Build history of the part. All positions in model axes, mm. Face numbers are marked on the shaded views. A direction names the side the tool comes from. Coordinates: 2 decimals unless noted, no trailing zeros. Order: outer loops, then holes, each group sorted by start corner. A loop starts at its lowest first (then second) coordinate and runs counter-clockwise, first axis right, second up. Notation, with made-up numbers: (81, 47.5) - (131, 47.5) arc R10 ccw to (131, 54.5) - close; hole circle Ø7 at (18.5, -19.75). An arc over 180 degrees is marked (long way). Answer as CSV lines item,"result". Start each with the question number.
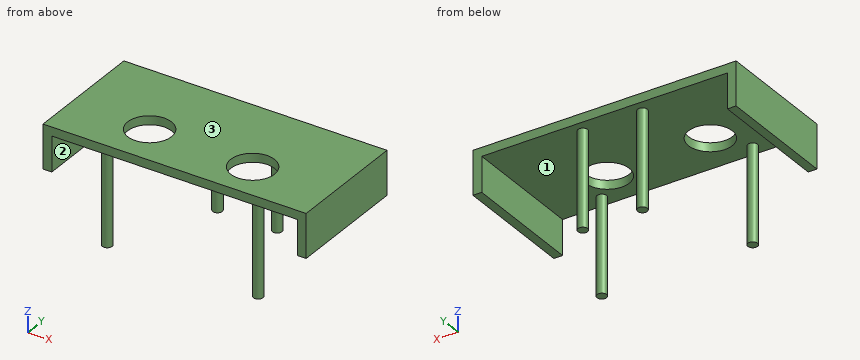
from build123d import *

# Parameters (mm, degrees)
ESQUISSE1_W             = 100
ESQUISSE1_H             = 69.87
BOSS_EXTRU_1_DEPTH      = 5
ESQUISSE2_R             = 12.5
ENL_V_MAT_EXTRU_1_DEPTH = 5
ESQUISSE3_W             = 25
ESQUISSE3_H             = 69.87
BOSS_EXTRU_2_DEPTH      = 5
ESQUISSE4_W             = 5
ESQUISSE4_H             = 69.87
BOSS_EXTRU_3_DEPTH      = 20
ESQUISSE2_3_R           = 2.75
BOSS_EXTRU_4_DEPTH      = 60
ESQUISSE2_4_R           = 2.75
BOSS_EXTRU_5_DEPTH      = 60
ESQUISSE2_5_R           = 2.75
BOSS_EXTRU_6_DEPTH      = 60
ESQUISSE2_6_R           = 2.75
BOSS_EXTRU_7_DEPTH      = 60


with BuildPart() as part:
    # Esquisse1 → Boss.-Extru.1 (new body)
    with BuildSketch(Plane.XY):
        with Locations((-50, 34.935)):
            Rectangle(ESQUISSE1_W, ESQUISSE1_H)
    extrude(amount=BOSS_EXTRU_1_DEPTH)

    # Esquisse2 → Enlèv. mat.-Extru.1 (cut)
    with BuildSketch(Plane.XY.offset(5)):
        with Locations((-80, 23.913092396)):
            Circle(ESQUISSE2_R)
        with Locations((-20, 21.980812212)):
            Circle(ESQUISSE2_R)
    extrude(amount=-ENL_V_MAT_EXTRU_1_DEPTH, mode=Mode.SUBTRACT)

    # Esquisse3 → Boss.-Extru.2 (add)
    with BuildSketch(Plane.XY.offset(5)):
        with Locations((-112.5, 34.935)):
            Rectangle(ESQUISSE3_W, ESQUISSE3_H)
        with Locations((12.5, 34.935)):
            Rectangle(ESQUISSE3_W, ESQUISSE3_H)
    extrude(amount=-BOSS_EXTRU_2_DEPTH)

    # Esquisse4 → Boss.-Extru.3 (add)
    with BuildSketch(Plane(origin=(0, 0, 0), x_dir=(-1, 0, 0), z_dir=(0, 0, -1))):
        with Locations((122.5, 34.935)):
            Rectangle(ESQUISSE4_W, ESQUISSE4_H)
        with Locations((-22.5, 34.935)):
            Rectangle(ESQUISSE4_W, ESQUISSE4_H)
    extrude(amount=BOSS_EXTRU_3_DEPTH)

    # Esquisse2<3> → Boss.-Extru.4 (add)
    with BuildSketch(Plane.XY.offset(5)):
        with Locations((-67, 62.87)):
            Circle(ESQUISSE2_3_R)
    extrude(amount=-BOSS_EXTRU_4_DEPTH)

    # Esquisse2<4> → Boss.-Extru.5 (add)
    with BuildSketch(Plane.XY.offset(5)):
        with Locations((-33, 62.87)):
            Circle(ESQUISSE2_4_R)
    extrude(amount=-BOSS_EXTRU_5_DEPTH)

    # Esquisse2<5> → Boss.-Extru.6 (add)
    with BuildSketch(Plane.XY.offset(5)):
        with Locations((-93, 7)):
            Circle(ESQUISSE2_5_R)
    extrude(amount=-BOSS_EXTRU_6_DEPTH)

    # Esquisse2<6> → Boss.-Extru.7 (add)
    with BuildSketch(Plane.XY.offset(5)):
        with Locations((-7, 7)):
            Circle(ESQUISSE2_6_R)
    extrude(amount=-BOSS_EXTRU_7_DEPTH)


solid = part.part
(1) Band-saw the part on B-B on z = -7.5. List the corners of the cut face in (x, y).
(2) Probe L1, parallel to Y at x = -80, z = 1; L2, parallel to X at y = 33, z = -11; L3, parallel to Y at x = -20, z = 1.55. List the from-to ranges inside material, lowest first. Write a range as [from, to].
(3) Band-saw the part on A-A on x = -80. List the corners of the cut face in (y, z), plus the area to 3 significant figures.
(4) Drop flat-ended pins along their axis: pin 1 Ø2 at (x, y) = (-59.5, 50) entering from -Z; pin 2 Ø8 at (y, z) = (16, -28) entering from -X; pin 3 Ø6 at (y, z) = (11.5, -23.5) entering from -X; pin 4 Ø5.5 at (x, y) = (-121.5, 31.5) entering from -Z. Give the stop position or say it passes through.
(5) Which spindle directions (+Z, -Z, +X, -X, +Y, -Y) get a long thin tool onto all of the face, cutting with end or side? Do the marked faces 1, 2 and 3. Say none if no direction does.
(6) Band-saw the part on C-C on y = 30. List the corners of the cut face in (x, z).
(7) Band-saw the part on D-D on y = 52.5. List the corners of the cut face in (x, z), plus the area to 3 significant figures.
Filled in:
1,outline,"(-125, 0) - (-120, 0) - (-120, 69.87) - (-125, 69.87) - close; circle Ø5.5 at (-93, 7); circle Ø5.5 at (-67, 62.87); circle Ø5.5 at (-33, 62.87); circle Ø5.5 at (-7, 7); (20, 0) - (25, 0) - (25, 69.87) - (20, 69.87) - close"
2,L1,"y = [0, 11.41], [36.41, 69.87]"
2,L2,"x = [-125, -120], [20, 25]"
2,L3,"y = [0, 9.48], [34.48, 69.87]"
3,outline,"(0, 0) - (11.41, 0) - (11.41, 5) - (0, 5) - close; (36.41, 0) - (69.87, 0) - (69.87, 5) - (36.41, 5) - close"
3,area,"224 mm^2"
4,pin 1,"stops at z = 0"
4,pin 2,"passes through"
4,pin 3,"stops at x = -95.3"
4,pin 4,"stops at z = -20"
5,face 1,"-Z"
5,face 2,"-Z, +Y, -Y"
5,face 3,"+Z, +X, -X, +Y, -Y"
6,outline,"(-125, -20) - (-120, -20) - (-120, 0) - (-90.92, 0) - (-90.92, 5) - (-125, 5) - close; (-69.08, 0) - (-29.59, 0) - (-29.59, 5) - (-69.08, 5) - close; (-10.41, 0) - (20, 0) - (20, -20) - (25, -20) - (25, 5) - (-10.41, 5) - close"
7,outline,"(-125, -20) - (-120, -20) - (-120, 0) - (20, 0) - (20, -20) - (25, -20) - (25, 5) - (-125, 5) - close"
7,area,"950 mm^2"
